Geometry: see drawing. Coordinates: mm, zero at the bounding-box minimum. Give positions to 0.01 mm unless a question says otherwise; leave off trailing zeros. Write each loop counter-clockwise with the first axis right and the second up, starting at its lowest first coordinate (ties: lowest second). Pieces come first, ordered by that corner, then holes. Notation, with made-up numbers: (87.25, 9.5) -> (138.25, 9.5) arc R23 cw to (138.25, 37.5) -> close; hole circle Ø4 at (42.5, 64.5). An arc over 180 degrees is marked (long way). Answer as a JSON object with one key per item and string values. Group by question number.
Item 1: Section query B-B on y = 44. Return the cut outline in (x, z) (1 decimal).
Item 2: First-contact query: pin 1 Ø3 at (x, y) = (3, 31) entering from +Z; pin 2 Ø1.9 at (x, y) = (4.76, 57.79) entering from -Z. Flat tips, straight axial feed; report the tip coordinate or a pass-through.
Item 3: Section query A-A on x = 7.75. Return the cut outline in (y, z) (1 decimal).
Item 4: Ray query, probe 1 along Y at (x, z) = (4.75, 7.25) (1 decimal); probe 2 along Z at (x, y) = (4.5, 38); probe 3 along Y at (x, z) = (5, 4) (1 decimal). Return the intervals inside material, ascending. Write a range as from..to.
Item 5: Section query C-C on z = 8.5. Return the cut outline in (x, y) (1 decimal).
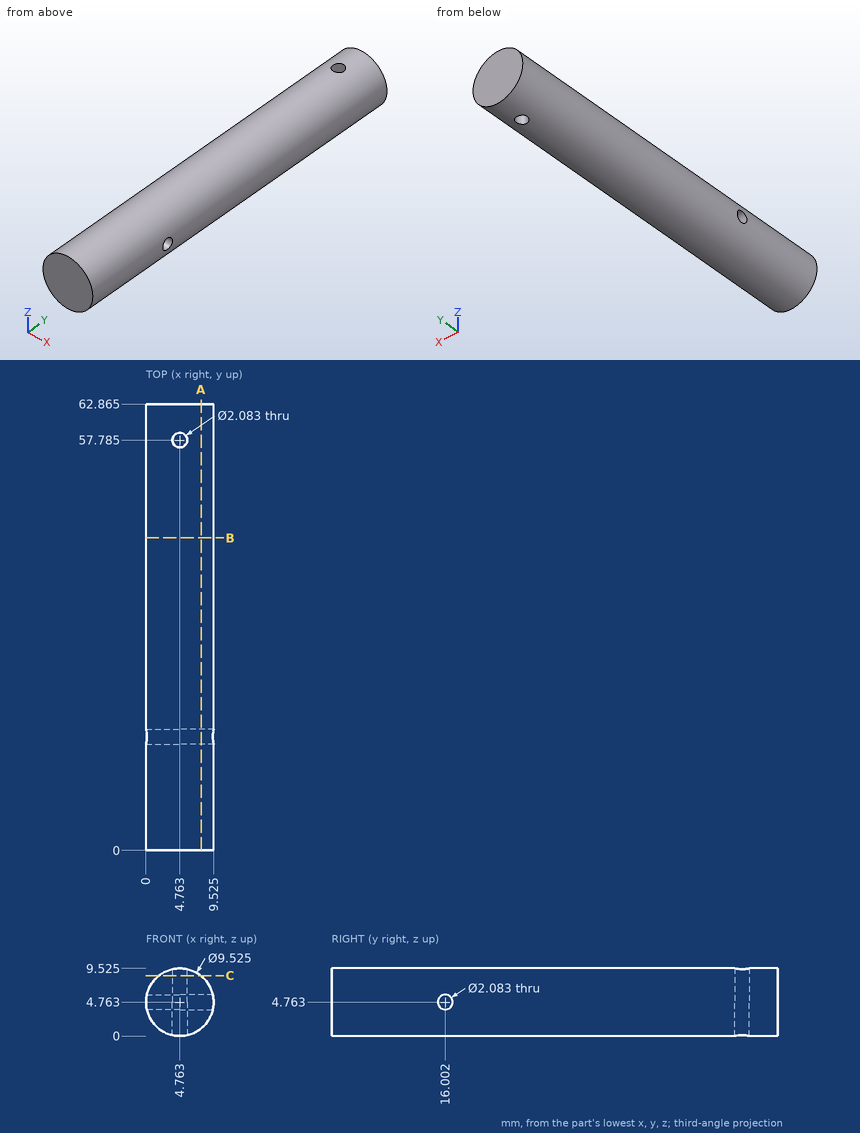
Worked answers:
{
 "1": {"outline": "circle Ø9.5 at (4.8, 4.8)"},
 "2": {"pin 1": "z = 9.52", "pin 2": "through"},
 "3": {"outline": "(0, 1.1) -> (62.9, 1.1) -> (62.9, 8.5) -> (0, 8.5) -> close; hole circle Ø2.1 at (16, 4.8)"},
 "4": {"probe 1": "0..56.7, 58.8..62.9", "probe 2": "0.01..9.52", "probe 3": "0..15.3, 16.7..56.8, 58.8..62.9"},
 "5": {"outline": "(1.8, 0) -> (7.7, 0) -> (7.7, 62.9) -> (1.8, 62.9) -> close; hole circle Ø2.1 at (4.8, 57.8)"}
}
